Read the model definition and answer for the solid it produces. Units are mm, in the model's axes. Face numbers are marked on the shaded views. A direction names the side the tool comes from. Coordinates: 2 decimals unless noted, no trailing zeros. Order: outer loops, then holes, each group sorted by start corner. A loop starts at its lowest first (then second) coordinate and runs counter-clockwise, first axis right, second up. Notation, with made-up numbers: (-27.5, 53.25) -> (3.5, 53.25) arc R9 cw to (3.5, 61.25) -> close; hole circle Ø1 at (19.5, 22.25). An arc over 180 degrees is marked (long way). Answer in a Markdown table with one row per item.
from build123d import *

# Parameters (mm, degrees)
ESQUISSE1_R             = 1
BOSS_EXTRU_1_DEPTH      = 1.5
CONG_1_R                = 2
CONG_2_R                = 1
ESQUISSE2_W             = 7
ESQUISSE2_H             = 2
BOSS_EXTRU_2_DEPTH      = 6.8
CONG_3_R                = 0.5
CONG_4_R                = 0.5
CONG_5_R                = 2
CONG_6_R                = 2
ESQUISSE3_R             = 1.5
ENL_V_MAT_EXTRU_1_DEPTH = 5
CONG_7_R                = 5
ENL_V_MAT_EXTRU_2_DEPTH = 7


with BuildPart() as part:
    # Esquisse1 → Boss.-Extru.1 (new body)
    with BuildSketch(Plane.XY):
        with BuildLine():
            Line((5.725874922, 0), (15.999999988, 0))
            ThreePointArc((15.999999988, 0), (18.000588979, 2.000588991), (15.999999988, 4.001177983))
            Line((15.999999988, 4.001177983), (13.999999884, 4.001177983))
            Line((13.999999884, 4.001177983), (22.919071704, 14.001177983))
            Line((22.919071704, 14.001177983), (28.487225861, 14.001177983))
            ThreePointArc((28.487225861, 14.001177983), (30.487225861, 16.001177983), (28.487225861, 18.001177983))
            Line((28.487225861, 18.001177983), (21.522063421, 18.001177983))
            Line((21.522063421, 18.001177983), (20.277949706, 22.137339224))
            ThreePointArc((20.277949706, 22.137339224), (17.786631004, 23.476492361), (16.447477867, 20.98517366))
            Line((16.447477867, 20.98517366), (17.053942849, 18.968929547))
            ThreePointArc((17.053942849, 18.968929547), (16.590729073, 12.03075257), (11.678911432, 7.108668233))
            Line((11.678911432, 7.108668233), (-3.597341835, 0.147035641))
            ThreePointArc((-3.597341835, 0.147035641), (-4.587900453, -2.502264951), (-1.938599861, -3.492823569))
            Line((-1.938599861, -3.492823569), (5.725874922, 0))
        make_face()
        with Locations((28.487225861, 16.001177983)):
            Circle(ESQUISSE1_R, mode=Mode.SUBTRACT)
        with Locations((15.999999988, 2.000588991)):
            Circle(ESQUISSE1_R, mode=Mode.SUBTRACT)
        with Locations((18.362713786, 21.561256442)):
            Circle(ESQUISSE1_R, mode=Mode.SUBTRACT)
        with Locations((-2.767970848, -1.672893964)):
            Circle(ESQUISSE1_R, mode=Mode.SUBTRACT)
    extrude(amount=BOSS_EXTRU_1_DEPTH)

    # Congé1
    cong_1_edges = [part.edges().sort_by_distance(p)[0] for p in [
        (21.522063421, 18.001177983, 0.75),
        (22.919071704, 14.001177983, 0.75),
    ]]
    fillet(cong_1_edges, radius=CONG_1_R)

    # Congé2
    cong_2_edges = [part.edges().sort_by_distance(p)[0] for p in [
        (13.999999884, 4.001177983, 0.75),
    ]]
    fillet(cong_2_edges, radius=CONG_2_R)

    # Esquisse2 → Boss.-Extru.2 (add)
    with BuildSketch(Plane(origin=(0, 0, 0), x_dir=(-1, 0, 0), z_dir=(0, 0, -1))):
        with Locations((-2.999999988, 1)):
            Rectangle(ESQUISSE2_W, ESQUISSE2_H)
    extrude(amount=-BOSS_EXTRU_2_DEPTH)

    # Congé3
    cong_3_edges = [part.edges().sort_by_distance(p)[0] for p in [
        (3.484354553, 2, 1.5),
    ]]
    fillet(cong_3_edges, radius=CONG_3_R)

    # Congé4
    cong_4_edges = [part.edges().sort_by_distance(p)[0] for p in [
        (-0.500000012, 0.779271889, 1.5),
    ]]
    fillet(cong_4_edges, radius=CONG_4_R)

    # Congé5
    cong_5_edges = [part.edges().sort_by_distance(p)[0] for p in [
        (6.499999988, 1.25, 1.5),
    ]]
    fillet(cong_5_edges, radius=CONG_5_R)

    # Congé6
    cong_6_edges = [part.edges().sort_by_distance(p)[0] for p in [
        (6.499999988, 1, 6.8),
        (-0.500000012, 1, 6.8),
    ]]
    fillet(cong_6_edges, radius=CONG_6_R)

    # Esquisse3 → Enlèv. mat.-Extru.1 (cut)
    with BuildSketch(Plane(origin=(0, 2, 0), x_dir=(1, 0, 0), z_dir=(0, 1, 0))):
        with Locations(Location((2.999999988, -4.3, 0), (0, 0, 270))):
            Circle(ESQUISSE3_R)
    extrude(amount=-ENL_V_MAT_EXTRU_1_DEPTH, mode=Mode.SUBTRACT)

    # Congé7
    cong_7_edges = [part.edges().sort_by_distance(p)[0] for p in [
        (5.725874922, 0, 0.75),
    ]]
    fillet(cong_7_edges, radius=CONG_7_R)

    # Esquisse4 → Enlèv. mat.-Extru.2 (cut)
    with BuildSketch(Plane(origin=(0, 0, 0), x_dir=(-1, 0, 0), z_dir=(0, 0, -1))):
        Polygon((0.500000012, 2), (-0.468709119, 2), (0.500000012, 1.558543777), align=None)
    extrude(amount=-ENL_V_MAT_EXTRU_2_DEPTH, mode=Mode.SUBTRACT)


solid = part.part
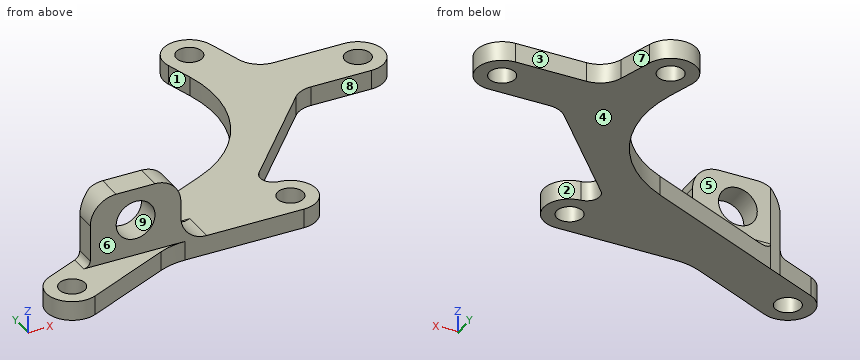
Q1. The part is cut by section C-C (y = 12). Write down the section's boundary in (x, z).
Outcome:
| item | result |
|---|---|
| outline | (16.58, 0) -> (21.13, 0) -> (21.13, 1.5) -> (16.58, 1.5) -> close |
Q2. The part is cut by section A-A (z = 4.3). Write down the section's boundary in (x, y), then the cut area to 3 significant figures.
Outcome:
| item | result |
|---|---|
| outline | (-0.5, 0) -> (1.5, 0) -> (1.5, 2) -> (0.47, 2) -> (-0.5, 1.56) -> close; (4.5, 0) -> (6.5, 0) -> (6.5, 2) -> (4.5, 2) -> close |
| area | 7.79 mm² |
Q3. For the marked faces 5, 6, 7, 8 and 9, determine the directions among +Z, -Z, +X, -X, +Y, -Y from which every point of the face is accessible in a straight line to the end or side of a thin tool.
Outcome:
| item | result |
|---|---|
| face 5 | +Z, +X, -X, +Y |
| face 6 | +Z, +X, -Y |
| face 7 | +Z, -Z, +X, +Y |
| face 8 | +Z, -Z, +X, -Y |
| face 9 | +Y, -Y |
Q4. Given pin 1 (1.2 mm diameter, centred on x = 26, z = 0.5, fed in from -Y); pin 2 (0.7 mm diameter, centred on y = 1, z = 4, fed in from +X); pin 3 (0.8 mm diameter, centred on y = 1, z = 3, fed in from -X), each flat-ended and moving along its own axis, determine where each tip first touches the part or whether it passes through.
Outcome:
| item | result |
|---|---|
| pin 1 | y = 14 |
| pin 2 | x = 6.5 |
| pin 3 | x = -0.5 |
Q5. The part is cut by section B-B (x = 3). Write down the section's boundary in (y, z).
Outcome:
| item | result |
|---|---|
| outline | (-1.24, 0) -> (3.15, 0) -> (3.15, 1.5) -> (2.5, 1.5) arc R0.5 cw to (2, 2) -> (2, 2.8) -> (0, 2.8) -> (0, 1.5) -> (-1.24, 1.5) -> close; (0, 5.8) -> (2, 5.8) -> (2, 6.8) -> (0, 6.8) -> close |
Q6. Consider line 1 (Y direction, x = 16, z = 0.65); line 2 (X direction, y = 1.35, z = 4.3); line 3 (Y direction, x = 4.5, z = 6). Determine where each line is inside the solid, lowest interval first.
Outcome:
| item | result |
|---|---|
| line 1 | 0 to 1, 3 to 4.02, 6.24 to 10.92 |
| line 2 | -0.5 to 1.5, 4.5 to 6.5 |
| line 3 | 0 to 2 |
Q7. For a pull along Y with two mould halves and no side action, classify the marked faces 1, 2, 3 and 4 as pulls with the +Y half, pulls with the -Y half, needs draft (parallel to the pull), parting line crosses it, or undercut.
Outcome:
| item | result |
|---|---|
| face 1 | undercut |
| face 2 | undercut |
| face 3 | pulls with the +Y half |
| face 4 | needs draft |
Q8. The part is cut by section D-D (z = 0.5). Give the number of separate pieces and of enclosed holes in the cut face, then the cut area to 3 significant figures.
Outcome:
| item | result |
|---|---|
| separate pieces | 1 |
| enclosed holes | 4 |
| area | 205 mm² |
